The listing builds one solid part. Answer for the finished solid, in the listing's coordinates (mm). A direction names the side the tool comes from. Give positions to 0.01 mm unless a question says otherwise; leave off trailing zeros. Order: outer loops, then holes, each group sorted by start corner. A loop starts at its lowest first (then second) coordinate and runs counter-clockwise, first axis right, second up. Notation, with made-up numbers: (45.25, 67.5) - (79.25, 67.5) arc R6 cw to (79.25, 78.5) - close; hole circle Ø5 at (51.25, 77.25). An arc over 180 degrees is marked (long way). Answer in a Markdown table with one row per item.
from build123d import *

# Parameters (mm, degrees)
F1_DEPTH = 2.54


with BuildPart() as f1:
    # F0 (on Right) → F1 (new body)
    with BuildSketch(Plane.YZ):
        Polygon((0, 0), (-35.532644, 0), (0, -76.2), align=None)
        with BuildLine():
            Line((-20.550144, -26.753266), (-14.061934, -26.753266))
            ThreePointArc((-14.061934, -26.753266), (-10.469832, -29.293266), (-6.877729, -26.753266))
            Line((-6.877729, -26.753266), (-0.389519, -26.753266))
            ThreePointArc((-0.389519, -26.753266), (-10.469832, -35.643266), (-20.550144, -26.753266))
        make_face(mode=Mode.SUBTRACT)
        with BuildLine():
            Line((-19.264794, -20.396594), (-8.621269, -1.993714))
            Line((-8.621269, -1.993714), (-1.285707, -1.993714))
            Line((-1.285707, -1.993714), (-9.052472, -15.422615))
            ThreePointArc((-9.052472, -15.422615), (-3.233258, -18.351814), (-0.389519, -24.213266))
            Line((-0.389519, -24.213266), (-6.877729, -24.213266))
            ThreePointArc((-6.877729, -24.213266), (-10.469832, -21.673266), (-14.061934, -24.213266))
            Line((-14.061934, -24.213266), (-20.550144, -24.213266))
            ThreePointArc((-20.550144, -24.213266), (-20.098474, -22.240605), (-19.264794, -20.396594))
        make_face(mode=Mode.SUBTRACT)
        Polygon((35.532644, 0), (0, 0), (0, -76.2), align=None)
        Polygon((0.862135, -1.993714), (7.959447, -1.993714), (20.32, -26.753266), (7.62, -26.753266), (7.62, -35.643266), (1.27, -35.643266), (1.27, -20.403266), (10.052618, -20.403266), align=None, mode=Mode.SUBTRACT)
    extrude(amount=-F1_DEPTH)


solid = f1.part
Item 1: Find section C-C on y = 12. Write down the section's boundary in (x, z), then the cut area to 3 significant figures.
Answer block:
| item | result |
|---|---|
| outline | (-2.54, -50.47) - (0, -50.47) - (0, -26.75) - (-2.54, -26.75) - close; (-2.54, -10.09) - (0, -10.09) - (0, 0) - (-2.54, 0) - close |
| area | 85.9 mm² |
Item 2: Find section D-D on y = -10.5. Write down the section's boundary in (x, z).
Answer block:
| item | result |
|---|---|
| outline | (-2.54, -53.68) - (0, -53.68) - (0, -35.64) - (-2.54, -35.64) - close; (-2.54, -29.29) - (0, -29.29) - (0, -21.67) - (-2.54, -21.67) - close; (-2.54, -5.24) - (0, -5.24) - (0, 0) - (-2.54, 0) - close |
Item 3: Which of the six approach directions +Z, -Z, +X, -X, +Y, -Y give full straight-line access (tool end or side, diameter ignored) to faces 5 (the face through (-1.25, 17.52, -38.63)), 6 (the face through (-1, 4, -35.643))?
Answer block:
| item | result |
|---|---|
| face 5 | -Z, +X, -X, +Y |
| face 6 | +X, -X |
Item 4: Determine the mould class of faces 1 (the face through (-1.3, -18, -37.6)), 2 (the face through (-1.25, -20.11, -22.27)), 3 (the face through (-1, -5, -1.994)), 4 (the face through (-2.54, 0, -29)) for opening direction Y: pulls with the +Y half, pulls with the -Y half, needs draft (parallel to the pull), parting line crosses it, or undercut.
Answer block:
| item | result |
|---|---|
| face 1 | pulls with the -Y half |
| face 2 | undercut |
| face 3 | undercut |
| face 4 | needs draft |
Item 5: Each of these flat-tipped pins is pushed along its axis until it touches: P1, Ø0.8, axis at x = -1.5, y = 3.5, coming from the -Z side; P2, Ø0.8, axis at x = -1.5, y = -17.5, coming from the -Z side; P3, Ø1.3, axis at x = -1, y = 4.5, coming from the -Z side. Where does it stop, or does it pass through?
Answer block:
| item | result |
|---|---|
| P1 | z = -69.55 |
| P2 | z = -39.53 |
| P3 | z = -67.94 |
Item 6: Find section A-A on x = -1.15. Write down the section's boundary in (y, z), then the cut area to 3 significant figures.
Answer block:
| item | result |
|---|---|
| outline | (-35.53, 0) - (0, -76.2) - (35.53, 0) - close; hole (-20.55, -26.75) arc R10.16 ccw to (-0.39, -26.75) - (-6.88, -26.75) arc R3.81 cw to (-14.06, -26.75) - close; hole (-20.55, -24.21) - (-14.06, -24.21) arc R3.81 cw to (-6.88, -24.21) - (-0.39, -24.21) arc R10.16 ccw to (-9.05, -15.42) - (-1.29, -1.99) - (-8.62, -1.99) - (-19.26, -20.4) arc R10.16 ccw to start; hole (0.86, -1.99) - (10.05, -20.4) - (1.27, -20.4) - (1.27, -35.64) - (7.62, -35.64) - (7.62, -26.75) - (20.32, -26.75) - (7.96, -1.99) - close |
| area | 2,060 mm² |
Item 7: Find section B-B on z = -10. Write down the section's boundary in (x, y).
Answer block:
| item | result |
|---|---|
| outline | (-2.54, -30.87) - (0, -30.87) - (0, -13.25) - (-2.54, -13.25) - close; (-2.54, -5.92) - (0, -5.92) - (0, 4.86) - (-2.54, 4.86) - close; (-2.54, 11.96) - (0, 11.96) - (0, 30.87) - (-2.54, 30.87) - close |
Item 8: Consider line 1 (Y direction, x = -1.8, z = -11); line 2 (Z direction, x = -1.85, y = 6); line 3 (Z direction, x = -0.6, y = -15). Determine where each line is inside the solid, lowest interval first.
Answer block:
| item | result |
|---|---|
| line 1 | -30.4 to -13.83, -6.49 to 5.36, 12.46 to 30.4 |
| line 2 | -63.33 to -35.64, -20.4 to -12.29, -1.99 to 0 |
| line 3 | -44.03 to -34.58, -26.75 to -24.21, -13.02 to 0 |
